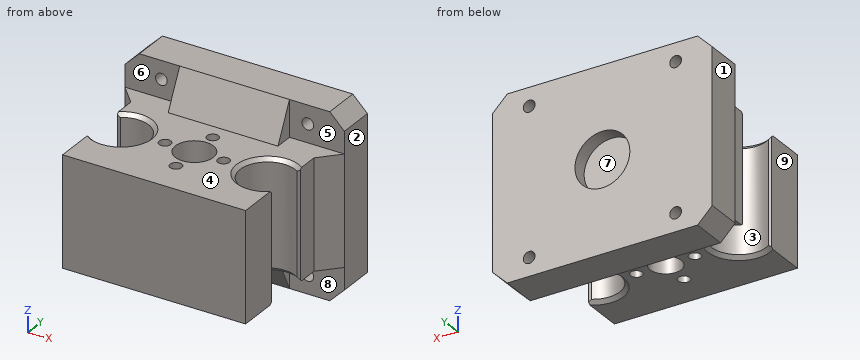
from build123d import *

# Parameters (mm, degrees)
SKETCH_1_W          = 50
SKETCH_1_H          = 35
EXTRUDE_1_DEPTH     = 30
HOLE_WIZARD_360_D   = 8.5
HOLE_WIZARD_465_D   = 3.2
HOLE_WIZARD_619_D   = 15
CHAMFER_1_SIZE      = 1
CHAMFER_1_SIZE_2    = 0.708203932
HOLE_WIZARD_1_D     = 10.4
HOLE_WIZARD_1_DEPTH = 11
SKETCH_11_W         = 60
SKETCH_11_H         = 50
EXTRUDE_3_DEPTH     = 10
HOLE_WIZARD_2_D     = 3.2
CHAMFER_2_SIZE      = 4
HOLE_WIZARD_3_D     = 15
HOLE_WIZARD_3_DEPTH = 4
EXTRUDE_4_DEPTH     = 15
RIB_22_REACH        = 49.762
SKETCH_19_WALL_W    = 104.820665624
SKETCH_19_WALL_H    = 30


with BuildPart() as part:
    # 草图1 → 凸台-拉伸1 (new body)
    with BuildSketch(Plane.XY):
        Rectangle(SKETCH_1_W, SKETCH_1_H)
    extrude(amount=EXTRUDE_1_DEPTH)

    # Hole Wizard 360 (through all)
    with Locations(Plane.XY.offset(30)):
        with Locations((0, 0)):
            Hole(HOLE_WIZARD_360_D / 2)

    # Hole Wizard 465 (through all)
    with Locations(Plane.XY.offset(30)):
        with Locations((8, 0), (0, 8), (-8, 0), (0, -8)):
            Hole(HOLE_WIZARD_465_D / 2)

    # Hole Wizard 619 (through all)
    with Locations(Plane.XY.offset(30)):
        with Locations((20, 0), (-20, 0)):
            Hole(HOLE_WIZARD_619_D / 2)

    # 倒角1
    # the kernel refuses this chamfer: 1, 0.708203932 mm, written as the material it takes off along each edge
    with BuildSketch(Plane(origin=(-20, 0, 0), x_dir=(-0.8790200859122482, 0.4767847402789059, 0), z_dir=(-0.4767847402789059, -0.8790200859122482, 0))) as chamfer_1_piece_1:
        Polygon((7.5, -CHAMFER_1_SIZE), (7.5 + CHAMFER_1_SIZE, 0), (7.5, 0), align=None)
    revolve(axis=Axis((-20, 0, 0), (0, 0, -1)), revolution_arc=303.048763938, mode=Mode.SUBTRACT)
    with BuildSketch(Plane(origin=(-20, 0, 30), x_dir=(-0.879020085912248, 0.47678474027890627, 0), z_dir=(-0.47678474027890627, -0.879020085912248, 0))) as chamfer_1_piece_2:
        Polygon((7.5 + CHAMFER_1_SIZE, 0), (7.5, CHAMFER_1_SIZE), (7.5, 0), align=None)
    revolve(axis=Axis((-20, 0, 30), (0, 0, -1)), revolution_arc=303.048763938, mode=Mode.SUBTRACT)
    with BuildSketch(Plane(origin=(20, 0, 30), x_dir=(0.879020085912248, -0.4767847402789061, 0), z_dir=(0.4767847402789061, 0.879020085912248, 0))) as chamfer_1_piece_3:
        Polygon((7.5 + CHAMFER_1_SIZE, 0), (7.5, CHAMFER_1_SIZE), (7.5, 0), align=None)
    revolve(axis=Axis((20, 0, 30), (0, 0, -1)), revolution_arc=303.048763938, mode=Mode.SUBTRACT)
    with BuildSketch(Plane(origin=(20, 0, 0), x_dir=(0.8790200859122481, 0.476784740278906, 0), z_dir=(0.476784740278906, -0.8790200859122481, 0))) as chamfer_1_piece_4:
        Polygon((7.5, CHAMFER_1_SIZE), (7.5 + CHAMFER_1_SIZE, 0), (7.5, 0), align=None)
    revolve(axis=Axis((20, 0, 0), (0, 0, 1)), revolution_arc=303.048763938, mode=Mode.SUBTRACT)
    with BuildSketch(Plane(origin=(-25, 5.590169944, 32.778051389), x_dir=(0.7914486393779661, 0.611235675682274, 0), z_dir=(0, 0, -1)), Plane(origin=(25, -5.590169944, 32.778051389), x_dir=(-0.7914486393779661, -0.611235675682274, 0), z_dir=(0, 0, -1))) as chamfer_1_piece_5:
        with BuildLine():
            Line((1.080663788, 0), (CHAMFER_1_SIZE_2 * 0.611235676113, -CHAMFER_1_SIZE_2 * 0.791448639936))
            Line((CHAMFER_1_SIZE_2 * 0.611235676113, -CHAMFER_1_SIZE_2 * 0.791448639936), (0, 0))
            ThreePointArc((0, 0), (0.555522087, -0.019473843), (1.080663788, 0))
        make_face()
    extrude(amount=35.556102778, mode=Mode.SUBTRACT)
    with BuildSketch(Plane(origin=(-25, -5.590169944, 32.778051389), x_dir=(0.7914486393779665, -0.6112356756822735, 0), z_dir=(0, 0, -1))) as chamfer_1_piece_6:
        with BuildLine():
            Line((1.080663788, 0), (CHAMFER_1_SIZE_2 * 0.611235676113, CHAMFER_1_SIZE_2 * 0.791448639936))
            Line((CHAMFER_1_SIZE_2 * 0.611235676113, CHAMFER_1_SIZE_2 * 0.791448639936), (0, 0))
            ThreePointArc((0, 0), (0.555522087, 0.019473843), (1.080663788, 0))
        make_face()
    extrude(amount=35.556102778, mode=Mode.SUBTRACT)
    with BuildSketch(Plane(origin=(25, 5.590169944, 32.778051389), x_dir=(0, 1, 0), z_dir=(0, 0, -1))) as chamfer_1_piece_7:
        with BuildLine():
            Line((CHAMFER_1_SIZE_2, 0), (0.660540261, -0.855289885))
            ThreePointArc((0.660540261, -0.855289885), (0.354967464, -0.427764092), (0, 0))
            Line((0, 0), (CHAMFER_1_SIZE_2, 0))
        make_face()
    extrude(amount=35.556102778, mode=Mode.SUBTRACT)

    # 孔1
    with Locations(Plane.XY.offset(30)):
        with Locations((0, 0)):
            Hole(HOLE_WIZARD_1_D / 2, depth=HOLE_WIZARD_1_DEPTH)

    # 草图11 → 凸台-拉伸3 (add)
    with BuildSketch(Plane(origin=(0, 17.5, 0), x_dir=(1, 0, 0), z_dir=(0, 1, 0))):
        with Locations((0, -15)):
            Rectangle(SKETCH_11_W, SKETCH_11_H)
    extrude(amount=EXTRUDE_3_DEPTH)

    # 孔2 (through all)
    with Locations(Plane(origin=(0, 27.5, 0), x_dir=(1, 0, 0), z_dir=(0, 1, 0))):
        with Locations((-20, 5), (20, 5), (20, -35), (-20, -35)):
            Hole(HOLE_WIZARD_2_D / 2)

    # 倒角2
    chamfer_2_edges = [part.edges().sort_by_distance(p)[0] for p in [
        (30, 22.5, 40),
        (30, 22.5, -10),
        (-30, 22.5, -10),
        (-30, 22.5, 40),
    ]]
    chamfer(chamfer_2_edges, length=CHAMFER_2_SIZE)

    # 孔3
    with Locations(Plane(origin=(0, 27.5, 0), x_dir=(1, 0, 0), z_dir=(0, 1, 0))):
        with Locations((0, -15)):
            Hole(HOLE_WIZARD_3_D / 2, depth=HOLE_WIZARD_3_DEPTH)

    # 草图16 → 凸台-拉伸4 (add, symmetric)
    with BuildSketch(Plane(origin=(0, 0, 0), x_dir=(0, 0, -1), z_dir=(1, 0, 0))):
        Polygon((-40, 17.5), (-30, 12.5), (-30, 17.5), align=None)
        Polygon((10, 17.5), (0, 17.5), (0, 12.5), align=None)
    extrude(amount=EXTRUDE_4_DEPTH, both=True)

    # 草图19 wall → 筋22 (add, up to next)
    with BuildSketch(Plane(origin=(-27.5, 14.843465885, 15), x_dir=(0.685325827281, -0.728236575888, 0), z_dir=(0.728236575888, 0.685325827281, 0)), mode=Mode.PRIVATE) as rib_22_sk1:
        Rectangle(SKETCH_19_WALL_W, SKETCH_19_WALL_H)
    rib_22_tool1 = extrude(rib_22_sk1.sketch, amount=RIB_22_REACH, mode=Mode.PRIVATE) - part.part
    rib_22 = rib_22_tool1.solids().sort_by_distance((-27.5, 14.843465885, 15))[0]
    add(rib_22)

    # 镜向1: 筋22 across plane
    add(rib_22.mirror(Plane(origin=(0, 0, 0), x_dir=(0, 0, 1), z_dir=(1, 0, 0))))


solid = part.part
Check sheet for the modelled part. Datum: model origin and axes. Units: mm. Face numbers are marked on the shaded views. A direction names the side the tool comes from. Coordinates: 2 decimals unless noted, no trailing zeros. Write each loop counter-clockwise with the first axis right and the second up, starting at its lowest first coordinate (ties: lowest second). Pieces come first, ordered by that corner, then holes. Notation, with made-up numbers: M 68.5,-13 L 112.5,-13 A18 cw 112.5,-7 Z; hole C 71.25,-1 d5. An arc over 180 degrees is marked long. Answer as CSV lines item,"result".
Q1. Cross-section at C-C (x = -20). Record the boundary of the cut face in (y, z), then the cut area to 3 significant figures.
Check result:
outline,"M -17.5,0 L -8.5,0 L -7.5,1 L -7.5,29 L -8.5,30 L -17.5,30 Z; M 7.5,1 L 8.5,0 L 17.5,0 L 17.5,-3.4 L 27.5,-3.4 L 27.5,33.4 L 17.5,33.4 L 17.5,30 L 8.5,30 L 7.5,29 Z; M 17.5,-10 L 27.5,-10 L 27.5,-6.6 L 17.5,-6.6 Z; M 17.5,36.6 L 27.5,36.6 L 27.5,40 L 17.5,40 Z"
area,"1,030 mm^2"
Q2. Cross-section at A-A (y = 0). Record the boundary of the cut face in (x, z).
Check result:
outline,"M -12.5,1 L -11.5,0 L -9.6,0 L -9.6,30 L -11.5,30 L -12.5,29 Z; M -6.4,0 L -4.25,0 L -4.25,19 L -5.2,19 L -5.2,30 L -6.4,30 Z; M 4.25,0 L 6.4,0 L 6.4,30 L 5.2,30 L 5.2,19 L 4.25,19 Z; M 9.6,0 L 11.5,0 L 12.5,1 L 12.5,29 L 11.5,30 L 9.6,30 Z"
Q3. Set-up check for the marked faces 5, 6, 7, 8 and 9: record each of +Z, -Z, +X, -X, +Y, -Y from which the full face is reachable in a straight line by a thin tool's end or side.
Check result:
face 5,"+Z, +X, -Y"
face 6,"+Z, -X, -Y"
face 7,"+Y"
face 8,"-Z, +X, -Y"
face 9,"+Z, -Z, -X, -Y"
Q4. Cross-section at B-B (z = -5). Record the boundary of the cut face in (x, y).
Check result:
outline,"M -30,17.5 L -21.6,17.5 L -21.6,27.5 L -30,27.5 Z; M -18.4,17.5 L -15,17.5 L -15,15 L 15,15 L 15,17.5 L 18.4,17.5 L 18.4,27.5 L -18.4,27.5 Z; M 21.6,17.5 L 30,17.5 L 30,27.5 L 21.6,27.5 Z"
Q5. Mould release check, pull along X, two halves, no side actions. Record for the marked faces 1, 2, 3 and 4: released by +X, released by -X, zero draft, split by the parting line, or undercut.
Check result:
face 1,"released by -X"
face 2,"released by +X"
face 3,"undercut"
face 4,"zero draft"
Q6. Cross-section at D-D (z = 26.5). Record the boundary of the cut face in (x, y).
Check result:
outline,"M -30,17.5 L -25,12.19 L -25,6.3 L -24.14,6.25 A7.5 cw long -24.14,-6.25 L -25,-6.3 L -25,-17.5 L 25,-17.5 L 25,-6.3 L 24.14,-6.25 A7.5 cw long 24.14,6.25 L 25,6.3 L 25,12.19 L 30,17.5 L 30,27.5 L -30,27.5 Z; hole C -8,0 d3.2; hole C 0,0 d10.4; hole C 0,-8 d3.2; hole C 0,8 d3.2; hole C 8,0 d3.2"
Q7. Go/stop test with flat-tipped pins: pin 1 (5 mm diameter, centred on x = 0, y = 8, fed in from -Z); pin 2 (2.5 mm diameter, centred on x = 0, y = -8, fed in from +Z); pin 3 (12.5 mm diameter, centred on y = -10.5, z = 8.5, fed in from -X); pin 4 (5 mm diameter, centred on x = -2.5, z = 15, fed in from +Y). Record where each tip stops, or that it passes through.
Check result:
pin 1,"z = 0"
pin 2,"through"
pin 3,"x = -25"
pin 4,"y = 23.5"
Q8. Material ranges on probe 1 along X at (y, z) = (23, -5); probe 2 along Z at (x, y) = (-20, 23); probe 3 along Y at (x, z) = (0, 13), recorded low to high. Write a range as from..to.
Check result:
probe 1,"-30..-21.6, -18.4..18.4, 21.6..30"
probe 2,"-10..-6.6, -3.4..33.4, 36.6..40"
probe 3,"-17.5..-9.6, -6.4..-4.25, 4.25..6.4, 9.6..23.5"
